Here's how the part is built. I have some questions about the finished solid (model axes, mm). A direction names the side the tool comes from. Round coordinates to 2 decimals unless told otherwise and drop trailing zeros. Write each loop counter-clockwise with the first axis right and the second up, starting at its lowest first coordinate (ties: lowest second). Pieces come first, ordered by that corner, then holes. Notation, with made-up numbers: M 24.5,-35.5 L 55.5,-35.5 A15 cw 55.5,-14.5 Z; hole C 89.5,-34 d9. An arc over 180 degrees is marked long. Use one line per item in the form item = value. Start each with the question number.
Q1. I want a section at C-C on z = 13. State how many separate pieces and enclosed holes the cut face has, and give its area (3 significant figures).
Q2. We'd pull the mould along Y, two halves only. Please class faces 1 (the face through (0, -28, 10)), 2 (the face through (71, 0, 10)), 3 (the face through (19, -19, 5.08)), 4 (the face through (108, -19, 5.08)): +Y half, -Y half, draft (parallel to the pull), parting line (faces both ways), or undercut.
Q3. I need wall thicknesses on line 1 along Y through (x, z) = (90.5, 17.5); line 2 along Y through (x, z) = (21, 15.25); line 3 along Z through (x, y) = (20, -21). Which ranges of each line are inside material? Lowest first, please. Write a range as from..to.
Q4. I'm going to push flat-ended pins straight in: pin 1 Ø4 at (x, y) = (34, -22) entering from +Z; pin 2 Ø10 at (x, z) = (102.5, 20.5) entering from -Y. Where does each tip first touch, or does it pass through?
Q5. For faces 5 (the face through (55, -19, 5.08)), 6 (the face through (142.3, -28.3, 22.8)), which set-ups out of +Z, -Z, +X, -X, +Y, -Y let a thin tool reach every point of the face, with its end or its side?
Q6. I want a section at B-B on x = 57. List the corners of the cut face in (y, z) for me.
```python
from build123d import *

# Parameters (mm, degrees)
F0_W     = 144.78
F0_H     = 55.88
F1_DEPTH = 25.4
F2_R     = 6.37356
F3_DEPTH = 20.32
F4_SIZE  = 5.08
F5_SIZE  = 5.08


with BuildPart() as f1:
    # F0 (on Top) → F1 (new body)
    with BuildSketch(Plane.XY):
        with Locations((72.39, -27.94)):
            Rectangle(F0_W, F0_H)
    extrude(amount=F1_DEPTH)

    # F2 (on face) → F3 (cut)
    with BuildSketch(Plane.XY.offset(25.4)):
        with Locations((125.770479, -18.998763)):
            Circle(F2_R)
        with Locations((125.770479, -36.789436)):
            Circle(F2_R)
        with Locations((107.979804, -36.989331)):
            Circle(F2_R)
        with Locations((107.979804, -18.998763)):
            Circle(F2_R)
        with Locations((90.189137, -18.998763)):
            Circle(F2_R)
        with Locations((90.189137, -36.789436)):
            Circle(F2_R)
        with Locations((72.398461, -36.789436)):
            Circle(F2_R)
        with Locations((72.398461, -19.19866)):
            Circle(F2_R)
        with Locations((54.60779, -19.19866)):
            Circle(F2_R)
        with Locations((54.60779, -36.789436)):
            Circle(F2_R)
        with Locations((36.817115, -36.789436)):
            Circle(F2_R)
        with Locations((36.817115, -18.998763)):
            Circle(F2_R)
        with Locations((19.02644, -18.998763)):
            Circle(F2_R)
        with Locations((19.02644, -36.789436)):
            Circle(F2_R)
    extrude(amount=-F3_DEPTH, mode=Mode.SUBTRACT)

    # F4
    f4_edges = [f1.edges().sort_by_distance(p)[0] for p in [
        (72.39, -55.88, 25.4),
        (72.39, 0, 25.4),
        (144.78, -27.94, 25.4),
        (0, -27.94, 25.4),
    ]]
    chamfer(f4_edges, length=F4_SIZE)

    # F5
    f5_edges = [f1.edges().sort_by_distance(p)[0] for p in [
        (144.78, -55.88, 10.16),
        (144.78, 0, 10.16),
        (0, -55.88, 10.16),
        (0, 0, 10.16),
    ]]
    chamfer(f5_edges, length=F5_SIZE)


solid = f1.part
```
Reported:
q1.separate_pieces = 1
q1.enclosed_holes = 14
q1.area = 6,250 mm^2
q2.face_1 = draft
q2.face_2 = +Y half
q2.face_3 = undercut
q2.face_4 = undercut
q3.line_1 = -55.88..-43.16, -30.42..-25.36, -12.63..0
q3.line_2 = -55.88..-42.85, -30.73..-25.06, -12.94..0
q3.line_3 = 0..5.08
q4.pin_1 = 5.08
q4.pin_2 = -55.88
q5.face_5 = +Z
q5.face_6 = +Z, +X, +Y, -Y
q6.outline = M -55.88,0 L 0,0 L 0,20.32 L -5.08,25.4 L -13.29,25.4 L -13.29,5.08 L -25.11,5.08 L -25.11,25.4 L -30.88,25.4 L -30.88,5.08 L -42.7,5.08 L -42.7,25.4 L -50.8,25.4 L -55.88,20.32 Z
